Geometry check sheet. Reference: the model listing, model coordinates, mm. Face numbers are marked on the shaded views. A direction names the side the tool comes from. Round coordinates to 2 decimals unless told otherwise and drop trailing zeros. Write each loop counter-clockwise with the first axis right and the second up, starting at its lowest first coordinate (ties: lowest second). Pieces come first, ordered by that corner, then holes. Notation, with made-up numbers: M 77,3 L 94,3 A18 cw 94,37 Z; hole C 62,84.25 d4. An arc over 180 degrees is marked long. One line per item, written item: value. Start each with the question number.
1. Scan lines: probe 1 along Y at (x, z) = (0, 3.25); probe 2 along X at (y, z) = (1.25, 4.25); probe 3 along Z at (x, y) = (-3, -3). Record each from-to range of solid material in increasing order. Write a range as [from, to].
2. Depth check by flat-ended pin: P1, Ø5, axis at x = 1, y = 2, coming from the +Z side; P2, Ø1.5, axis at x = 2.5, z = 4, coming from the -Y side; P3, Ø1, axis at y = 0, z = 3.5, coming from the +X side; P4, Ø1.5, axis at y = 0.5, z = 4, coming from the -X side. Enter the tip coordinate at first touch or a pass-through.
3. Access from +Z, -Z, +X, -X, +Y, -Y to the whole of each face (thin tool, end or side, straight path). Record for the marked faces 1 and 2.
4. Section check A-A (x = 0). Record the boundary of the cut face in (y, z) (3 decimals), and give its area (3 significant figures).
5. Release check for a two-part mould opening along Y. For the marked faces 3, 4 and 5 record: pulls with the +Y half, pulls with the -Y half, needs draft (parallel to the pull), parting line crosses it, or undercut.
6. Section check C-C (z = 4.45). Record the boundary of the cut face in (x, y), and give its area (3 significant figures).
from build123d import *

# Parameters (mm, degrees)
F0_R     = 3.95
F0_R_2   = 2.95
F1_DEPTH = 5.4
F0_R_3   = 5.075
F2_DEPTH = 2
F3_R     = 0.75


with BuildPart() as f1:
    # F0 (on Top) → F1 (new body)
    with BuildSketch(Plane.XY):
        Circle(F0_R)
        Circle(F0_R_2, mode=Mode.SUBTRACT)
    extrude(amount=F1_DEPTH)

    # F0 (on Top) → F2 (join)
    with BuildSketch(Plane.XY):
        Circle(F0_R_3)
        Circle(F0_R, mode=Mode.SUBTRACT)
    extrude(amount=F2_DEPTH)

    # F3
    f3_edges = [f1.edges().sort_by_distance(p)[0] for p in [
        (-5.075, 0, 0),
        (-2.95, 0, 0),
    ]]
    fillet(f3_edges, radius=F3_R)


solid = f1.part
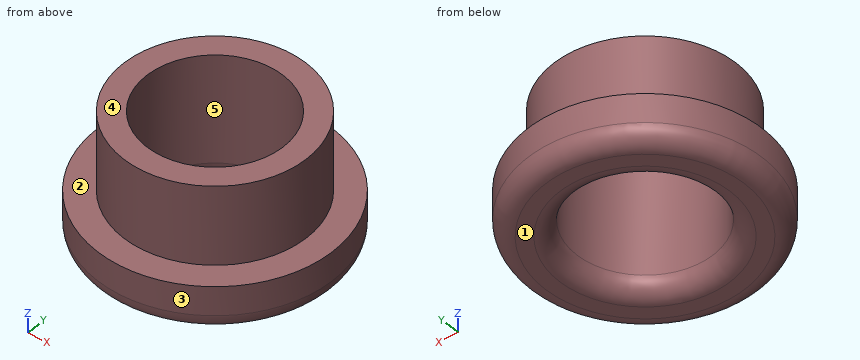
Result sheet:
1. probe 1: y = [-3.95, -2.95], [2.95, 3.95]
1. probe 2: x = [-3.75, -2.67], [2.67, 3.75]
1. probe 3: z = [0, 2]
2. P1: stops at z = 5.4
2. P2: stops at y = -3.54
2. P3: stops at x = 3.95
2. P4: stops at x = -3.95
3. face 1: -Z, +X, -X, +Y, -Y
3. face 2: +Z
4. outline: M -5.075,0.75 A0.75 ccw -4.325,0 L -3.7,0 A0.75 ccw -2.95,0.75 L -2.95,5.4 L -3.95,5.4 L -3.95,2 L -5.075,2 Z; M 2.95,0.75 A0.75 ccw 3.7,0 L 4.325,0 A0.75 ccw 5.075,0.75 L 5.075,2 L 3.95,2 L 3.95,5.4 L 2.95,5.4 Z
4. area: 14.8 mm2
5. face 3: parting line crosses it
5. face 4: needs draft
5. face 5: undercut
6. outline: C 0,0 d7.9; hole C 0,0 d5.9
6. area: 21.7 mm2
